Can you work these out from the model? Positions are in its coordinate system, mm. Face numbers are marked on the shaded views. Round coordinates to 2 decimals unless told otherwise and drop trailing zeros. Answer as a JSON object with one key per item and string values. Group by question number.
from build123d import *

# Parameters (mm, degrees)
F0_R     = 3.81
F1_DEPTH = 25.4


with BuildPart() as f1:
    # F0 (on Front) → F1 (new body)
    with BuildSketch(Plane.XZ):
        with BuildLine():
            Line((8.163403, 9.728764), (8.622894, 10.991205))
            ThreePointArc((8.622894, 10.991205), (8.047978, 11.418886), (7.451888, 11.816525))
            Line((7.451888, 11.816525), (6.417451, 10.959303))
            ThreePointArc((6.417451, 10.959303), (7.316343, 10.380805), (8.163403, 9.728764))
        make_face()
        with BuildLine():
            ThreePointArc((9.910585, 7.941681), (9.081062, 8.878306), (8.163403, 9.728764))
            ThreePointArc((8.163403, 9.728764), (7.316343, 10.380805), (6.417451, 10.959303))
            ThreePointArc((6.417451, 10.959303), (5.526004, 11.43474), (4.599586, 11.837813))
            ThreePointArc((4.599586, 11.837813), (3.556733, 12.191786), (2.487134, 12.454082))
            ThreePointArc((2.487134, 12.454082), (1.249631, 12.638371), (0, 12.7))
            ThreePointArc((0, 12.7), (-1.068009, 12.655013), (-2.128452, 12.520371))
            ThreePointArc((-2.128452, 12.520371), (-3.116945, 12.311566), (-4.085712, 12.024847))
            ThreePointArc((-4.085712, 12.024847), (-5.112114, 11.625674), (-6.100074, 11.13908))
            ThreePointArc((-6.100074, 11.13908), (-7.166515, 10.484801), (-8.163402, 9.728765))
            ThreePointArc((-8.163402, 9.728765), (-8.952628, 9.0078), (-9.678428, 8.223018))
            ThreePointArc((-9.678428, 8.223018), (-10.30144, 7.427673), (-10.85926, 6.585322))
            ThreePointArc((-10.85926, 6.585322), (-11.388945, 5.619779), (-11.83299, 4.611978))
            ThreePointArc((-11.83299, 4.611978), (-12.22937, 3.425277), (-12.507058, 2.205332))
            ThreePointArc((-12.507058, 2.205332), (-12.648213, 1.145737), (-12.69976, 0.078024))
            ThreePointArc((-12.69976, 0.078024), (-12.665777, -0.93171), (-12.551639, -1.935548))
            ThreePointArc((-12.551639, -1.935548), (-12.336763, -3.015672), (-12.029119, -4.07312))
            ThreePointArc((-12.029119, -4.07312), (-11.569966, -5.236973), (-10.998523, -6.35))
            ThreePointArc((-10.998523, -6.35), (-10.425558, -7.252429), (-9.778733, -8.103479))
            ThreePointArc((-9.778733, -8.103479), (-9.103656, -8.855136), (-8.370967, -9.550754))
            ThreePointArc((-8.370967, -9.550754), (-7.512072, -10.240057), (-6.596689, -10.852359))
            ThreePointArc((-6.596689, -10.852359), (-5.496847, -11.448785), (-4.343656, -11.934096))
            ThreePointArc((-4.343656, -11.934096), (-3.324669, -12.257103), (-2.282129, -12.493274))
            ThreePointArc((-2.282129, -12.493274), (-1.281833, -12.635146), (-0.273426, -12.697056))
            ThreePointArc((-0.273426, -12.697056), (0.827601, -12.673006), (1.922405, -12.553659))
            ThreePointArc((1.922405, -12.553659), (3.148308, -12.303583), (4.343655, -11.934096))
            ThreePointArc((4.343655, -11.934096), (5.331869, -11.526542), (6.28231, -11.037327))
            ThreePointArc((6.28231, -11.037327), (7.139774, -10.50303), (7.952054, -9.902264))
            ThreePointArc((7.952054, -9.902264), (8.78003, -9.176114), (9.541984, -8.380963))
            ThreePointArc((9.541984, -8.380963), (10.320335, -7.401398), (10.998522, -6.35))
            ThreePointArc((10.998522, -6.35), (11.493567, -5.402584), (11.907185, -4.416892))
            ThreePointArc((11.907185, -4.416892), (12.220601, -3.45643), (12.456679, -2.474093))
            ThreePointArc((12.456679, -2.474093), (12.624186, -1.385616), (12.696763, -0.286721))
            ThreePointArc((12.696763, -0.286721), (12.699191, -0.143369), (12.7, 0))
            ThreePointArc((12.7, 0), (12.651673, 1.106878), (12.507059, 2.205331))
            ThreePointArc((12.507059, 2.205331), (12.277297, 3.249303), (11.960557, 4.270256))
            ThreePointArc((11.960557, 4.270256), (11.583274, 5.207472), (11.132686, 6.111734))
            ThreePointArc((11.132686, 6.111734), (10.561344, 7.053226), (9.910585, 7.941681))
        make_face()
        Circle(F0_R, mode=Mode.SUBTRACT)
        with BuildLine():
            Line((11.183078, 8.372554), (9.910585, 7.941681))
            ThreePointArc((9.910585, 7.941681), (10.561344, 7.053226), (11.132686, 6.111734))
            Line((11.132686, 6.111734), (12.018204, 7.122055))
            ThreePointArc((12.018204, 7.122055), (11.617479, 7.758549), (11.183078, 8.372554))
        make_face()
        with BuildLine():
            ThreePointArc((2.487134, 12.454082), (3.556733, 12.191786), (4.599586, 11.837813))
            Line((4.599586, 11.837813), (4.62851, 13.180963))
            ThreePointArc((4.62851, 13.180963), (3.912406, 13.410965), (3.184961, 13.602093))
            Line((3.184961, 13.602093), (2.487134, 12.454082))
        make_face()
        with BuildLine():
            Line((13.303993, 4.262002), (11.960557, 4.270256))
            ThreePointArc((11.960557, 4.270256), (12.277297, 3.249303), (12.507059, 2.205331))
            Line((12.507059, 2.205331), (13.670531, 2.877062))
            ThreePointArc((13.670531, 2.877062), (13.505027, 3.574234), (13.303993, 4.262002))
        make_face()
        with BuildLine():
            ThreePointArc((-2.128452, 12.520371), (-1.068009, 12.655013), (0, 12.7))
            Line((0, 12.7), (-0.459491, 13.962441))
            ThreePointArc((-0.459491, 13.962441), (-1.17481, 13.920514), (-1.887038, 13.841965))
            Line((-1.887038, 13.841965), (-2.128452, 12.520371))
        make_face()
        with BuildLine():
            ThreePointArc((-6.100074, 11.13908), (-5.112114, 11.625674), (-4.085712, 12.024847))
            Line((-4.085712, 12.024847), (-4.926916, 13.072353))
            ThreePointArc((-4.926916, 13.072353), (-5.623325, 12.788241), (-6.303435, 12.467061))
            Line((-6.303435, 12.467061), (-6.100074, 11.13908))
        make_face()
        with BuildLine():
            Line((13.948509, -0.774596), (12.696763, -0.286721))
            ThreePointArc((12.696763, -0.286721), (12.624186, -1.385616), (12.456679, -2.474093))
            Line((12.456679, -2.474093), (13.784447, -2.269342))
            ThreePointArc((13.784447, -2.269342), (13.886604, -1.524178), (13.948509, -0.774596))
        make_face()
        with BuildLine():
            ThreePointArc((-9.678428, 8.223018), (-8.952628, 9.0078), (-8.163402, 9.728765))
            Line((-8.163402, 9.728765), (-9.326875, 10.400496))
            ThreePointArc((-9.326875, 10.400496), (-9.847891, 9.90858), (-10.342999, 9.390595))
            Line((-10.342999, 9.390595), (-9.678428, 8.223018))
        make_face()
        with BuildLine():
            Line((12.931012, -5.286759), (11.907185, -4.416892))
            ThreePointArc((11.907185, -4.416892), (11.493567, -5.402584), (10.998522, -6.35))
            Line((10.998522, -6.35), (12.321574, -6.58329))
            ThreePointArc((12.321574, -6.58329), (12.642924, -5.942842), (12.931012, -5.286759))
        make_face()
        with BuildLine():
            ThreePointArc((-11.83299, 4.611978), (-11.388945, 5.619779), (-10.85926, 6.585322))
            Line((-10.85926, 6.585322), (-12.176983, 6.847043))
            ThreePointArc((-12.176983, 6.847043), (-12.52784, 6.181757), (-12.842383, 5.498553))
            Line((-12.842383, 5.498553), (-11.83299, 4.611978))
        make_face()
        with BuildLine():
            Line((10.187277, -9.559304), (9.541984, -8.380963))
            ThreePointArc((9.541984, -8.380963), (8.78003, -9.176114), (7.952054, -9.902264))
            Line((7.952054, -9.902264), (9.100794, -10.598889))
            ThreePointArc((9.100794, -10.598889), (9.658033, -10.093725), (10.187277, -9.559304))
        make_face()
        with BuildLine():
            ThreePointArc((-12.69976, 0.078024), (-12.648213, 1.145737), (-12.507058, 2.205332))
            Line((-12.507058, 2.205332), (-13.83011, 1.972043))
            ThreePointArc((-13.83011, 1.972043), (-13.913034, 1.26031), (-13.959355, 0.545262))
            Line((-13.959355, 0.545262), (-12.69976, 0.078024))
        make_face()
        with BuildLine():
            Line((6.507467, -12.361787), (6.28231, -11.037327))
            ThreePointArc((6.28231, -11.037327), (5.331869, -11.526542), (4.343655, -11.934096))
            Line((4.343655, -11.934096), (5.207216, -12.963248))
            ThreePointArc((5.207216, -12.963248), (5.865056, -12.679196), (6.507467, -12.361787))
        make_face()
        with BuildLine():
            ThreePointArc((-12.029119, -4.07312), (-12.336763, -3.015672), (-12.551639, -1.935548))
            Line((-12.551639, -1.935548), (-13.729304, -2.582075))
            ThreePointArc((-13.729304, -2.582075), (-13.570439, -3.31724), (-13.372238, -4.042789))
            Line((-13.372238, -4.042789), (-12.029119, -4.07312))
        make_face()
        with BuildLine():
            Line((1.659305, -13.871107), (1.922405, -12.553659))
            ThreePointArc((1.922405, -12.553659), (0.827601, -12.673006), (-0.273426, -12.697056))
            Line((-0.273426, -12.697056), (0.158778, -13.969098))
            ThreePointArc((0.158778, -13.969098), (0.910361, -13.940306), (1.659305, -13.871107))
        make_face()
        with BuildLine():
            ThreePointArc((-9.778733, -8.103479), (-10.425558, -7.252429), (-10.998523, -6.35))
            Line((-10.998523, -6.35), (-11.862084, -7.379151))
            ThreePointArc((-11.862084, -7.379151), (-11.468114, -7.977672), (-11.043974, -8.555205))
            Line((-11.043974, -8.555205), (-9.778733, -8.103479))
        make_face()
        with BuildLine():
            Line((-2.960995, -13.652597), (-2.282129, -12.493274))
            ThreePointArc((-2.282129, -12.493274), (-3.324669, -12.257103), (-4.343656, -11.934096))
            Line((-4.343656, -11.934096), (-4.343656, -13.277558))
            ThreePointArc((-4.343656, -13.277558), (-3.657136, -13.482813), (-2.960995, -13.652597))
        make_face()
        with BuildLine():
            ThreePointArc((-6.596689, -10.852359), (-7.512072, -10.240057), (-8.370967, -9.550754))
            Line((-8.370967, -9.550754), (-8.857532, -10.80301))
            ThreePointArc((-8.857532, -10.80301), (-8.263279, -11.264063), (-7.645074, -11.692465))
            Line((-7.645074, -11.692465), (-6.596689, -10.852359))
        make_face()
    extrude(amount=F1_DEPTH)


solid = f1.part
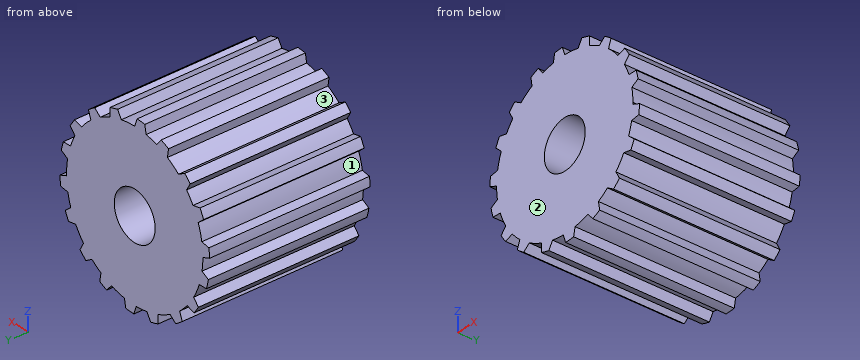
Item 1: If we mould it in two halves opening along X, with no side actions, what happens to the marked faces 1, 2 and 3? For each: +X half, -X half, draft (parallel to the pull), parting line (faces both ways), or undercut.
Item 2: I need wall thicknesses on line 1 (X direction, y = -23, z = -0.25); line 2 (X direction, y = -2, z = 12.75); line 3 (X direction, y = -12.25, z = 0.75). Which ranges of each line are inside material? Lowest first, please.
Item 3: I'm going to push a flat-ended pin straight in: pin 1 Ø1 at (y, z) = (-15.5, 4) entering from -X. Where does the tip first touch, or does it pass through?
Computed:
{
 "1": {"face 1": "-X half", "face 2": "draft", "face 3": "undercut"},
 "2": {"line 1": "x = -12.7 to -3.8, 3.8 to 12.7", "line 2": "x = -5.71 to -4.67, -2.09 to -0.02, 2.67 to 4.62", "line 3": "x = -13.95 to -3.74, 3.74 to 12.68"},
 "3": {"pin 1": "stops at x = -12.21"}
}
